```python
from build123d import *

# Parameters (mm, degrees)
SALIENTE_EXTRUIR1_DEPTH = 5
REDONDEO1_R             = 10
CROQUIS2_R              = 1.5
CORTAR_EXTRUIR1_DEPTH   = 135.669558943
CROQUIS4_W              = 80
CROQUIS4_H              = 50
CORTAR_EXTRUIR2_DEPTH   = 135.669558943
REDONDEO2_R             = 5
CROQUIS5_W              = 4
CROQUIS5_H              = 14.636342218
CORTAR_EXTRUIR3_DEPTH   = 135.669558943


with BuildPart() as part:
    # Croquis1 → Saliente-Extruir1 (new body)
    with BuildSketch(Plane(origin=(0, 0, 0), x_dir=(1, 0, 0), z_dir=(0, 1, 0))):
        Polygon((-88.1, 42.318171109), (88.1, 42.318171109), (108.1, 22.318171109), (127.75, 22.318171109), (127.75, 7.681828891), (105.75, 7.681828891), (77.75, -42.318171109), (-77.75, -42.318171109), (-105.75, 7.681828891), (-127.75, 7.681828891), (-127.75, 22.318171109), (-108.1, 22.318171109), align=None)
    extrude(amount=SALIENTE_EXTRUIR1_DEPTH)

    # Redondeo1
    redondeo1_edges = [part.edges().sort_by_distance(p)[0] for p in [
        (-88.1, 2.5, -42.318171109),
        (88.1, 2.5, -42.318171109),
        (108.1, 2.5, -22.318171109),
        (105.75, 2.5, -7.681828891),
        (77.75, 2.5, 42.318171109),
        (-77.75, 2.5, 42.318171109),
        (-105.75, 2.5, -7.681828891),
        (-108.1, 2.5, -22.318171109),
    ]]
    fillet(redondeo1_edges, radius=REDONDEO1_R)

    # Croquis2 → Cortar-Extruir1 (cut, through all)
    with BuildSketch(Plane(origin=(0, 5, 0), x_dir=(1, 0, 0), z_dir=(0, 1, 0))):
        with Locations(Location((70, -17.318171109, 0), (0, 0, 270))):
            Circle(CROQUIS2_R)
        with Locations(Location((-70, -17.318171109, 0), (0, 0, 270))):
            Circle(CROQUIS2_R)
        with Locations(Location((-119.996067812, 15, 0), (0, 0, 270))):
            Circle(CROQUIS2_R)
        with Locations(Location((119.996067812, 15, 0), (0, 0, 270))):
            Circle(CROQUIS2_R)
        with Locations(Location((-75, 32.318171109, 0), (0, 0, 270))):
            Circle(CROQUIS2_R)
        with Locations(Location((75, 32.318171109, 0), (0, 0, 270))):
            Circle(CROQUIS2_R)
        with Locations(Location((-17.5, -17.318171109, 0), (0, 0, 270))):
            Circle(CROQUIS2_R)
        with Locations(Location((17.5, -17.318171109, 0), (0, 0, 270))):
            Circle(CROQUIS2_R)
        with Locations(Location((-17.5, -37.318171109, 0), (0, 0, 270))):
            Circle(CROQUIS2_R)
        with Locations(Location((17.5, -37.318171109, 0), (0, 0, 270))):
            Circle(CROQUIS2_R)
    extrude(amount=-CORTAR_EXTRUIR1_DEPTH, mode=Mode.SUBTRACT)

    # Croquis4 → Cortar-Extruir2 (cut, through all)
    with BuildSketch(Plane(origin=(0, 5, 0), x_dir=(1, 0, 0), z_dir=(0, 1, 0))):
        with Locations((0, -17.318171109)):
            Rectangle(CROQUIS4_W, CROQUIS4_H)
    extrude(amount=-CORTAR_EXTRUIR2_DEPTH, mode=Mode.SUBTRACT)

    # Redondeo2
    redondeo2_edges = [part.edges().sort_by_distance(p)[0] for p in [
        (40, 2.5, 42.318171109),
        (-40, 2.5, 42.318171109),
        (-40, 2.5, -7.681828891),
        (40, 2.5, -7.681828891),
    ]]
    fillet(redondeo2_edges, radius=REDONDEO2_R)

    # Croquis5 → Cortar-Extruir3 (cut, through all)
    with BuildSketch(Plane(origin=(0, 5, 0), x_dir=(1, 0, 0), z_dir=(0, 1, 0))):
        with Locations((-125.75, 15)):
            Rectangle(CROQUIS5_W, CROQUIS5_H)
        with Locations((125.75, 15)):
            Rectangle(CROQUIS5_W, CROQUIS5_H)
    extrude(amount=-CORTAR_EXTRUIR3_DEPTH, mode=Mode.SUBTRACT)


solid = part.part
```
Model file for the job. Use its own axes, mm. A direction names the side the tool comes from. Coordinates: 2 decimals unless noted, no trailing zeros. Write each loop counter-clockwise with the first axis right and the second up, starting at its lowest first coordinate (ties: lowest second). Pieces come first, ordered by that corner, then holes. Notation, with made-up numbers: (33.5, -25.75) - (51.5, -25.75) arc R25 ccw to (51.5, 0.25) - close; hole circle Ø2 at (-27, -23.5). An arc over 180 degrees is marked (long way). One line per item, written item: value. Start each with the question number.
1. Slice it at B-B (z = 12.5). Write the cut outline in (x, y), plus the area to 3 significant figures.
2. Tool access for faces 1 (the flat face through (-118, 2, -7.682)), 2 (the cylindrical face through (-41.5, 2.46, 40.89)), 3 (the flat face through (118, 2, -22.318)): list every direction of +Z, -Z, +X, -X, +Y, -Y with a clear straight run to the whole face (end or side of a thin tool).
3. Probe line 1 (X direction, y = 1.25, z = -15); line 2 (Z direction, x = 70, y = 1.55); line 3 (Z direction, x = 2.5, y = 1.1). List the from-to ranges inside material, lowest first. Write a range as from..to.
4. Flat gauge pins, fed straight in: pin 1 (2.5 mm diameter, centred on x = -118, y = 2.5, fed in from -Z); pin 2 (2.5 mm diameter, centred on y = 2, z = 11.5, fed in from -X); pin 3 (1.5 mm diameter, centred on x = 119, y = 2.5, fed in from +Z); pin 4 (3 mm diameter, centred on x = 18, z = -11.5, fed in from -Y). Where does each tip first touch, or does it go through?
5. Mould opens along X. For faces 4 (the cylindrical face through (38.496, 2.465, -6.256)), 5 (the flat face through (-123.75, 3, -15)), 6 (the cylindrical face through (108.365, 2.535, -23.101)) say: released by +X, released by -X, zero draft, split by the parting line, or undercut.
6. Slice it at A-A (z = 0). Write the cut outline in (x, y).
Answers below:
1. outline: (-94.45, 0) - (-40, 0) - (-40, 5) - (-94.45, 5) - close; (40, 0) - (94.45, 0) - (94.45, 5) - (40, 5) - close
1. area: 544 mm^2
2. face 1: +Z, -X, +Y, -Y
2. face 2: +Z, +Y, -Y
2. face 3: -Z, +X, +Y, -Y
3. line 1: x = -123.75..-121.5, -118.5..118.5, 121.5..123.75
3. line 2: z = -42.32..15.82, 18.82..42.32
3. line 3: z = -42.32..-7.68
4. pin 1: stops at z = -22.32
4. pin 2: stops at x = -95.71
4. pin 3: stops at z = -7.68
4. pin 4: stops at y = 0
5. face 4: undercut
5. face 5: released by -X
5. face 6: released by +X
6. outline: (-101.45, 0) - (-40, 0) - (-40, 5) - (-101.45, 5) - close; (40, 0) - (101.45, 0) - (101.45, 5) - (40, 5) - close
